Check sheet for the modelled part. Datum: model origin and axes. Units: mm. A direction names the side the tool comes from. Give positions to 0.01 mm unless a question says otherwise; leave off trailing zeros. Write each loop counter-clockwise with the first axis right and the second up, starting at its lowest first coordinate (ties: lowest second). Pieces come first, ordered by that corner, then holes. Notation, with made-up numbers: (84, -7) -> (93, -7) arc R25 cw to (93, 17) -> close; hole circle Ø5 at (22, -35). An arc over 180 degrees is marked (long way). Use a Markdown table: item, result. Add a question column.
1. Scan lines: probe 1 along Y at (x, z) = (-2, 8.9); probe 2 along Z at (x, y) = (2, 17.5); probe 3 along Y at (x, z) = (-1.5, 9.6). Record each from-to range of solid material in increasing order. Write a range as [from, to].
2. Set-up check for faces 5 (the cylindrical face through (-31.4, -14, 9.1)), 6 (the cylindrical face through (-22.81, -16.26, 10.59)), 7 (the cylindrical face through (5.13, 15.682, 9.113)): record each of +Z, -Z, +X, -X, +Y, -Y from which the full face is reachable in a straight line by a thin tool's end or side.
3. Release check for a two-part mould opening along Y. For faces 1 (the flat face through (8.64, -2.49, 9.11)), 2 (the flat face through (0.5, 9, 9)), 3 (the flat face through (0, 1, 10)), 4 (the flat face through (0, -21, 9)) record: released by +Y, released by -Y, zero draft, split by the parting line, or undercut.
4. Cross-section at D-D (y = -14.5). Enter the section's corners in (x, z).
5. Cross-section at C-C (y = 12). Enter the section's corners in (x, z).
6. Cross-section at B-B (x = -13.5). Enter the section's corners in (y, z).
7. Gauge pin test, flat ends, axial feed: P1, Ø0.5, axis at y = 8.5, z = 9, coming from the +X side; P2, Ø4, axis at x = 6, y = 28.5, coming from the +Z side; P3, Ø1, axis at x = 11, y = -2, coming from the +Z side. Record the tip position at first contact, or that the pin passes through.
8. Cross-section at A-A (x = 14.5). Enter the section's corners in (y, z), then the cut area to 3 significant figures.
from build123d import *

# Parameters (mm, degrees)
SKETCH2_R           = 18
BOSS_EXTRUDE1_DEPTH = 1.8
BOSS_EXTRUDE7_START = -1.8
BOSS_EXTRUDE7_DEPTH = 1.8
SKETCH17_R          = 0.7
BOSS_EXTRUDE9_DEPTH = 1.8
BOSS_EXTRUDE2_START = -1.8
SKETCH3_R           = 35
SKETCH3_R_2         = 18
BOSS_EXTRUDE2_DEPTH = 1.8
SKETCH4_R           = 2.9
BOSS_EXTRUDE3_DEPTH = 3
SKETCH6_R           = 5
BOSS_EXTRUDE4_DEPTH = 1
SKETCH7_R           = 59.131365533
CUT_EXTRUDE1_DEPTH  = 10
FILLET1_R           = 6


with BuildPart() as part:
    # Sketch2 → Boss-Extrude1 (new body)
    with BuildSketch(Plane.XY.offset(10)):
        Circle(SKETCH2_R)
        with BuildLine():
            ThreePointArc((0, 0.538550206), (0.166421166, 0.512191682), (0.316551869, 0.435696269))
            Line((0.316551869, 0.435696269), (9.992349289, 13.753288904))
            ThreePointArc((9.992349289, 13.753288904), (13.753288904, 9.992349289), (16.167960777, 5.253288904))
            Line((16.167960777, 5.253288904), (0.512191682, 0.166421166))
            ThreePointArc((0.512191682, 0.166421166), (0.538550206, 0), (0.512191682, -0.166421166))
            Line((0.512191682, -0.166421166), (16.167960777, -5.253288904))
            ThreePointArc((16.167960777, -5.253288904), (13.753288904, -9.992349289), (9.992349289, -13.753288904))
            Line((9.992349289, -13.753288904), (0.316551869, -0.435696269))
            ThreePointArc((0.316551869, -0.435696269), (0.166421166, -0.512191682), (0, -0.538550206))
            Line((0, -0.538550206), (0, -17))
            ThreePointArc((0, -17), (-5.253288904, -16.167960777), (-9.992349289, -13.753288904))
            Line((-9.992349289, -13.753288904), (-0.316551869, -0.435696269))
            ThreePointArc((-0.316551869, -0.435696269), (-0.435696269, -0.316551869), (-0.512191682, -0.166421166))
            Line((-0.512191682, -0.166421166), (-16.167960777, -5.253288904))
            ThreePointArc((-16.167960777, -5.253288904), (-17, 0), (-16.167960777, 5.253288904))
            Line((-16.167960777, 5.253288904), (-0.512191682, 0.166421166))
            ThreePointArc((-0.512191682, 0.166421166), (-0.435696269, 0.316551869), (-0.316551869, 0.435696269))
            Line((-0.316551869, 0.435696269), (-9.992349289, 13.753288904))
            ThreePointArc((-9.992349289, 13.753288904), (-5.253288904, 16.167960777), (0, 17))
            Line((0, 17), (0, 0.538550206))
        make_face(mode=Mode.SUBTRACT)
        with BuildLine():
            Line((0.5, 1.198581445), (0.5, 16.492422502))
            ThreePointArc((0.5, 16.492422502), (5.193820321, 15.661233364), (9.454148381, 13.522909391))
            Line((9.454148381, 13.522909391), (0.5, 1.198581445))
        make_face(mode=Mode.SUBTRACT)
        with BuildLine():
            Line((-9.939558578, 13.170238239), (-0.985410197, 0.845910294))
            Line((-0.985410197, 0.845910294), (-15.530717393, 5.57196709))
            ThreePointArc((-15.530717393, 5.57196709), (-13.289739299, 9.779203923), (-9.939558578, 13.170238239))
        make_face(mode=Mode.SUBTRACT)
        with BuildLine():
            Line((-15.597133416, -5.383254519), (-1.109016994, -0.675780132))
            Line((-1.109016994, -0.675780132), (-10.098511219, -13.048757457))
            ThreePointArc((-10.098511219, -13.048757457), (-13.40733091, -9.617352956), (-15.597133416, -5.383254519))
        make_face(mode=Mode.SUBTRACT)
        with BuildLine():
            ThreePointArc((9.289494224, -13.636542709), (5.003553098, -15.723054932), (0.3, -16.497272502))
            Line((0.3, -16.497272502), (0.3, -1.263565384))
            Line((0.3, -1.263565384), (9.289494224, -13.636542709))
        make_face(mode=Mode.SUBTRACT)
        with BuildLine():
            Line((15.782543612, -4.812620609), (1.294427191, -0.105146222))
            Line((1.294427191, -0.105146222), (15.839734388, 4.620910574))
            ThreePointArc((15.839734388, 4.620910574), (16.499696789, -0.100029399), (15.782543612, -4.812620609))
        make_face(mode=Mode.SUBTRACT)
    extrude(amount=-BOSS_EXTRUDE1_DEPTH)

    # Sketch11 → Boss-Extrude7 (add)
    with BuildSketch(Plane(origin=(0, 0, 8.2), x_dir=(-1, 0, 0), z_dir=(0, 0, -1)).offset(BOSS_EXTRUDE7_START)):
        with BuildLine():
            ThreePointArc((-0.512191682, 0.166421166), (-0.435696269, 0.316551869), (-0.316551869, 0.435696269))
            Line((-0.316551869, 0.435696269), (-9.992349289, 13.753288904))
            ThreePointArc((-9.992349289, 13.753288904), (-13.753288904, 9.992349289), (-16.167960777, 5.253288904))
            Line((-16.167960777, 5.253288904), (-0.512191682, 0.166421166))
        make_face()
        with BuildLine():
            Line((0, 17), (0, 0.538550206))
            ThreePointArc((0, 0.538550206), (0.166421166, 0.512191682), (0.316551869, 0.435696269))
            Line((0.316551869, 0.435696269), (9.992349289, 13.753288904))
            ThreePointArc((9.992349289, 13.753288904), (5.253288904, 16.167960777), (0, 17))
        make_face()
        with BuildLine():
            Line((16.167960777, 5.253288904), (0.512191682, 0.166421166))
            ThreePointArc((0.512191682, 0.166421166), (0.531919759, 0.084247813), (0.538550206, 0))
            ThreePointArc((0.538550206, 0), (0.531919759, -0.084247813), (0.512191682, -0.166421166))
            Line((0.512191682, -0.166421166), (16.167960777, -5.253288904))
            ThreePointArc((16.167960777, -5.253288904), (17, 0), (16.167960777, 5.253288904))
        make_face()
        with BuildLine():
            Line((9.992349289, -13.753288904), (0.316551869, -0.435696269))
            ThreePointArc((0.316551869, -0.435696269), (0.166421166, -0.512191682), (0, -0.538550206))
            Line((0, -0.538550206), (0, -17))
            ThreePointArc((0, -17), (5.253288904, -16.167960777), (9.992349289, -13.753288904))
        make_face()
        with BuildLine():
            ThreePointArc((-0.316551869, -0.435696269), (-0.435696269, -0.316551869), (-0.512191682, -0.166421166))
            Line((-0.512191682, -0.166421166), (-16.167960777, -5.253288904))
            ThreePointArc((-16.167960777, -5.253288904), (-13.753288904, -9.992349289), (-9.992349289, -13.753288904))
            Line((-9.992349289, -13.753288904), (-0.316551869, -0.435696269))
        make_face()
        with BuildLine():
            ThreePointArc((0.316551869, 0.435696269), (0.166421166, 0.512191682), (0, 0.538550206))
            ThreePointArc((0, 0.538550206), (-0.166421166, 0.512191682), (-0.316551869, 0.435696269))
            ThreePointArc((-0.316551869, 0.435696269), (-0.435696269, 0.316551869), (-0.512191682, 0.166421166))
            ThreePointArc((-0.512191682, 0.166421166), (-0.538550206, 0), (-0.512191682, -0.166421166))
            ThreePointArc((-0.512191682, -0.166421166), (-0.435696269, -0.316551869), (-0.316551869, -0.435696269))
            ThreePointArc((-0.316551869, -0.435696269), (-0.166421166, -0.512191682), (0, -0.538550206))
            ThreePointArc((0, -0.538550206), (0.166421166, -0.512191682), (0.316551869, -0.435696269))
            ThreePointArc((0.316551869, -0.435696269), (0.435696269, -0.316551869), (0.512191682, -0.166421166))
            ThreePointArc((0.512191682, -0.166421166), (0.531919759, -0.084247813), (0.538550206, 0))
            ThreePointArc((0.538550206, 0), (0.531919759, 0.084247813), (0.512191682, 0.166421166))
            ThreePointArc((0.512191682, 0.166421166), (0.435696269, 0.316551869), (0.316551869, 0.435696269))
        make_face()
    extrude(amount=BOSS_EXTRUDE7_DEPTH)

    # Sketch17 → Boss-Extrude9 (add)
    with BuildSketch(Plane(origin=(0, 0, 8.2), x_dir=(-1, 0, 0), z_dir=(0, 0, -1))):
        Circle(SKETCH17_R)
    extrude(amount=-BOSS_EXTRUDE9_DEPTH)

    # Sketch3 → Boss-Extrude2 (add)
    with BuildSketch(Plane(origin=(0, 0, 8.2), x_dir=(-1, 0, 0), z_dir=(0, 0, -1)).offset(BOSS_EXTRUDE2_START)):
        Circle(SKETCH3_R)
        Circle(SKETCH3_R_2, mode=Mode.SUBTRACT)
    extrude(amount=BOSS_EXTRUDE2_DEPTH)

    # Sketch4 → Boss-Extrude3 (add)
    with BuildSketch(Plane(origin=(0, 0, 8.2), x_dir=(-1, 0, 0), z_dir=(0, 0, -1))):
        with Locations((0, 29)):
            Circle(SKETCH4_R)
        with Locations((25.11473671, -14.5)):
            Circle(SKETCH4_R)
        with Locations((-25.11473671, -14.5)):
            Circle(SKETCH4_R)
    extrude(amount=-BOSS_EXTRUDE3_DEPTH)

    # Sketch6 → Boss-Extrude4 (add)
    with BuildSketch(Plane(origin=(0, 0, 10), x_dir=(-1, 0, 0), z_dir=(0, 0, -1))):
        with Locations((0, 30)):
            Circle(SKETCH6_R)
        with Locations((25.980762114, -15)):
            Circle(SKETCH6_R)
        with Locations((-25.980762114, -15)):
            Circle(SKETCH6_R)
    extrude(amount=BOSS_EXTRUDE4_DEPTH)

    # Sketch7 → Cut-Extrude1 (cut)
    with BuildSketch(Plane(origin=(0, 0, 8.2), x_dir=(-1, 0, 0), z_dir=(0, 0, -1))):
        Circle(SKETCH7_R)
        Polygon((0, 42), (-36.373066959, -21), (36.373066959, -21), align=None, mode=Mode.SUBTRACT)
    extrude(amount=-CUT_EXTRUDE1_DEPTH, mode=Mode.SUBTRACT)

    # Fillet1
    fillet1_edges = [part.edges().sort_by_distance(p)[0] for p in [
        (4.186533479, 34.748711306, 9.1),
        (32.186533479, -13.748711306, 9.1),
        (28, -21, 9.1),
        (-28, -21, 9.1),
        (-32.186533479, -13.748711306, 9.1),
        (-4.186533479, 34.748711306, 9.1),
    ]]
    fillet(fillet1_edges, radius=FILLET1_R)


solid = part.part
Worked answers:
| question | item | result |
|---|---|---|
| 1 | probe 1 | y = [-21, -1.9], [-0.97, 1.18], [2.24, 34.82] |
| 1 | probe 2 | z = [8.2, 10] |
| 1 | probe 3 | y = [-21, -1.21], [-0.8, 1.01], [1.55, 34.92] |
| 2 | face 5 | +Z, -Z, -X |
| 2 | face 6 | +Z |
| 2 | face 7 | +Z, -Z |
| 3 | face 1 | undercut |
| 3 | face 2 | undercut |
| 3 | face 3 | zero draft |
| 3 | face 4 | released by -Y |
| 4 | outline | (-31.38, 8.2) -> (0.3, 8.2) -> (0.3, 10) -> (-22.21, 10) -> (-22.21, 11.2) -> (-28.01, 11.2) -> (-28.01, 10) -> (-31.38, 10) -> close; (7.87, 8.2) -> (31.38, 8.2) -> (31.38, 10) -> (28.01, 10) -> (28.01, 11.2) -> (22.21, 11.2) -> (22.21, 10) -> (7.87, 10) -> close |
| 5 | outline | (-17.32, 8.2) -> (-11.32, 8.2) -> (-11.32, 10) -> (-17.32, 10) -> close; (-9.09, 8.2) -> (0.5, 8.2) -> (0.5, 10) -> (-9.09, 10) -> close; (8.35, 8.2) -> (17.32, 8.2) -> (17.32, 10) -> (8.35, 10) -> close |
| 6 | outline | (-21, 8.2) -> (-9.49, 8.2) -> (-9.49, 10) -> (-21, 10) -> close; (-4.7, 8.2) -> (4.91, 8.2) -> (4.91, 10) -> (-4.7, 10) -> close; (9.49, 8.2) -> (18.62, 8.2) -> (18.62, 10) -> (9.49, 10) -> close |
| 7 | P1 | stops at x = 19.49 |
| 7 | P2 | stops at z = 10 |
| 7 | P3 | passes through |
| 8 | outline | (-21, 8.2) -> (-4.4, 8.2) -> (-4.4, 10) -> (-21, 10) -> close; (4.19, 8.2) -> (16.89, 8.2) -> (16.89, 10) -> (4.19, 10) -> close |
| 8 | area | 52.7 mm² |
